Autodesk Inventor part; units mm, degrees
ref_plane "作業平面1" through (28.1996, -140.8267, 0) normal (-1, 0, 0) x (0, 0, 1)
ref_plane "作業平面2" through (-116.8004, -45.8267, 0) normal (0, 1, 0) x (1, 0, 0)
ref_plane "YZ Plane" through (0, 0, 0) normal (1, 0, 0) x (0, 1, 0)
sketch "スケッチ1" plane through (0, 0, 0) normal (0, 0, 1) x (1, 0, 0)
  line L0 (-116.8004, 49.1733) -> (173.1996, 49.1733)
  line L1 (173.1996, 49.1733) -> (173.1996, -140.8267)
  line L2 (173.1996, -140.8267) -> (-116.8004, -140.8267)
  line L3 (-116.8004, -140.8267) -> (-116.8004, 49.1733)
  point P0 (0, 0)
  dimension "d0" = 290
  dimension "d1" = 190
extrude "押し出し1" add sketch "スケッチ1" along normal blind 15
sketch "スケッチ2" plane through (0, 0, 15) normal (0, 0, 1) x (1, 0, 0)
  line L0 (-111.8004, 42.1733) -> (163.1996, 42.1733)
  line L1 (163.1996, 42.1733) -> (163.1996, -133.8267)
  line L2 (163.1996, -133.8267) -> (-111.8004, -133.8267)
  line L3 (-111.8004, -133.8267) -> (-111.8004, 42.1733)
  line L4 (-111.8004, 27.1733) -> (-99.8004, 27.1733)
  line L5 (-99.8004, 27.1733) -> (-99.8004, 42.1733)
  line L6 (-116.8004, 49.1733) -> (-116.8004, -140.8267)
  line L7 (-116.8004, -140.8267) -> (173.1996, -140.8267)
  line L8 (173.1996, 49.1733) -> (-116.8004, 49.1733)
  line L9 (28.1996, -45.8267) -> (-116.8004, -45.8267)
  line L10 (28.1996, -45.8267) -> (28.1996, 49.1733)
  line L11 (168.1996, 27.1733) -> (158.1996, 27.1733)
  line L12 (158.1996, 27.1733) -> (158.1996, 42.1733)
  line L13 (-111.8004, -118.8267) -> (-99.8004, -118.8267)
  line L14 (-99.8004, -118.8267) -> (-99.8004, -133.8267)
  line L15 (158.1996, -118.8267) -> (158.1996, -133.8267)
  line L16 (168.1996, -118.8267) -> (158.1996, -118.8267)
  line L17 (-99.8004, 27.1733) -> (-99.8004, -118.8267)
  line L18 (158.1996, 27.1733) -> (151.1996, 27.1733)
  line L19 (151.1996, 27.1733) -> (151.1996, 42.1733)
  line L20 (158.1996, -118.8267) -> (151.1996, -118.8267)
  line L21 (151.1996, -118.8267) -> (151.1996, -133.8267)
  point P0 (0, 0)
  point P1 (163.1996, -118.8267)
  point P2 (163.1996, 27.1733)
  point P3 (158.1996, 42.1733)
  point P4 (-111.8004, -118.8267)
  point P5 (158.1996, -133.8267)
  dimension "d4" = 15
  dimension "d5" = 275
  dimension "d6" = 5
  dimension "d7" = 7
  dimension "d8" = 7
  dimension "d9" = 12
  dimension "d15" = 7
ref_plane "作業平面1" through (28.1996, -140.8267, 0) normal (-1, 0, 0) x (0, 0, 1)
ref_plane "作業平面2" through (-116.8004, -45.8267, 0) normal (0, 1, 0) x (1, 0, 0)
extrude "押し出し2" cut sketch "スケッチ2" against normal blind 8 contours L0 L10 L9 L17 L5 | L0 L19 L18 L11 L1 L16 L20 L21 L2 L14 L17 L9 L10 | L21 L20 L15 L2
sketch "スケッチ3" plane through (-116.8004, -140.8267, 0) normal (0, -1, 0) x (1, 0, 0)
  line L0 (275, 15) -> (275, 7)
  line L1 (275, 7) -> (17, 7)
  line L2 (275, 7) -> (270, 7)
  line L3 (270, 7) -> (270, 15)
  line L4 (0, 15) -> (290, 15)
  line L5 (270, 7) -> (270, 0)
  line L6 (290, 0) -> (0, 0)
  line L7 (275, 15) -> (275, 7)
  line L8 (275, 0) -> (275, 7)
  point P0 (116.8004, 0)
  dimension "d12" = 5
extrude "押し出し3" cut sketch "スケッチ3" against normal blind 7
sketch "スケッチ4" plane through (0, 0, 15) normal (0, 0, 1) x (1, 0, 0)
  circle A0 centre (-106.8004, 39.1733) radius 2.25
  circle A1 centre (163.1996, 39.1733) radius 2.25
  circle A2 centre (163.1996, -130.8267) radius 2.25
  line L0 (153.1996, -133.8267) -> (-99.8004, -133.8267)
  line L1 (-99.8004, -133.8267) -> (-99.8004, 42.1733)
  line L2 (-99.8004, 42.1733) -> (151.1996, 42.1733)
  line L3 (151.1996, 42.1733) -> (151.1996, 27.1733)
  line L4 (151.1996, 27.1733) -> (163.1996, 27.1733)
  line L5 (163.1996, 27.1733) -> (163.1996, -118.8267)
  line L6 (163.1996, -118.8267) -> (158.1996, -118.8267)
  line L7 (158.1996, -118.8267) -> (158.1996, -140.8267)
  line L8 (-116.8004, -140.8267) -> (153.1996, -140.8267)
  line L9 (173.1996, -140.8267) -> (173.1996, 49.1733)
  line L10 (173.1996, 49.1733) -> (-116.8004, 49.1733)
  line L11 (-116.8004, 49.1733) -> (-116.8004, -140.8267)
  line L12 (158.1996, -140.8267) -> (173.1996, -140.8267)
  circle A3 centre (-106.8004, -130.8267) radius 2.25
  line L13 (153.1996, -140.8267) -> (153.1996, -133.8267)
  point P0 (0, 0)
hole "穴1" at (-106.8004, 39.1733, 15) at (-106.8004, -130.8267, 15) at (163.1996, -130.8267, 15) at (163.1996, 39.1733, 15) direction (0, 0, -1) diameter 4.2 depth 4
fillet "フィレット2" radius 7 3 edges at (-99.8004, 42.1733, 11) (-99.8004, -133.8267, 11) (151.1996, 42.1733, 11)
fillet "フィレット3" radius 5 4 edges at (151.1996, 27.1733, 11) (163.1996, 27.1733, 11) (158.1996, -118.8267, 11) (163.1996, -118.8267, 11)
sketch "スケッチ5" plane through (0, 0, 0) normal (0, 0, -1) x (-1, 0, 0)
  line L0 (-143.1996, 41.1733) -> (92.8004, 41.1733)
  line L1 (92.8004, -133.8267) -> (-143.1996, -133.8267)
  line L2 (99.8004, 34.1733) -> (99.8004, -126.8267)
  line L3 (-163.1996, 22.1733) -> (-163.1996, -113.8267)
  line L4 (-173.1996, -140.8267) -> (-173.1996, 49.1733)
  line L5 (-28.1996, 87.1733) -> (-28.1996, -178.8267)
  line L6 (-231.1996, -45.8267) -> (174.8004, -45.8267)
  line L7 (-173.1996, 49.1733) -> (116.8004, 49.1733)
  point P0 (0, 0)
  point P1 (-98.1996, 41.6733)
  point P2 (41.8004, 41.6733)
  point P3 (-98.1996, -133.3267)
  point P4 (41.8004, -133.3267)
  point P5 (-165.6996, -30.8267)
  point P6 (-165.6996, -60.8267)
  point P7 (109.3004, -30.8267)
  point P8 (109.3004, -60.8267)
  point P9 (-68.1996, 41.6733)
  point P10 (11.8004, 41.6733)
  point P11 (-68.1996, -133.3267)
  point P12 (11.8004, -133.3267)
  dimension "d26" = 75
  dimension "d27" = 7.5
  dimension "d28" = 15
  dimension "d29" = 7.5
  dimension "d30" = 30
  dimension "d31" = 7.5
hole "穴2" at (98.1996, 41.6733, 0) at (-41.8004, 41.6733, 0) at (98.1996, -133.3267, 0) at (-41.8004, -133.3267, 0) at (165.6996, -30.8267, 0) at (165.6996, -60.8267, 0) at (-109.3004, -30.8267, 0) at (-109.3004, -60.8267, 0) at (68.1996, 41.6733, 0) at (-11.8004, 41.6733, 0) at (68.1996, -133.3267, 0) at (-11.8004, -133.3267, 0) direction (0, 0, 1) diameter 4.2 depth 4
properties part number "iPadHolder"
For this review, take the finished solid that the model builds, in its own axes (mm). A direction names the side the tool comes from. Give positions to 0.01 mm unless a question says otherwise; leave off trailing zeros. Write each loop counter-clockwise with the first axis right and the second up, starting at its lowest first coordinate (ties: lowest second). Pieces come first, ordered by that corner, then holes. Notation, with made-up numbers: M 86.25,-5 L 123.25,-5 A16 cw 123.25,7 Z; hole C -13,33 d5. An arc over 180 degrees is marked long. Answer as a JSON object with one key per item and string values. Group by question number.
Item 1: Draft analysis for pull direction X (two halves, no side actions). For faces 1 (the flat face through (-116.8, -47, 7)), 2 (the flat face through (26, -44, 0)), 3 (the flat face through (153.2, -137, 7)), state which applies: +X half, -X half, draft (parallel to the pull), parting line (faces both ways), or undercut.
Item 2: Tool access review of faces 4 (the flat face through (32, -133.827, 11)), 5 (the flat face through (158.2, -134, 9)), 6 (the flat face through (6, 46, 15)): name each direction out of +Z, -Z, +X, -X, +Y, -Y from which nothing blocks a thin tool from reaching the whole face with its end or side.
Item 3: For probe 1 along Y at (x, z) = (-42, 13); probe 2 along X at (y, z) = (6, 9.25); probe 3 along Y at (x, z) = (66.5, 3.25), list the stretches that pass through material, from the lowest coordinate up. Write a range as [from, to].
Item 4: Consider section A-A on x = 15. Write out the cut boundary in (y, z), plus the area to 3 significant figures.
Item 5: For pin 1 Ø4 at (x, y) = (65, -6) entering from -Z; pin 2 Ø3.5 at (x, y) = (98.2, -133.33) entering from -Z; pin 3 Ø8 at (x, y) = (-73.5, -85.5) entering from +Z; pin 4 Ø2 at (x, y) = (-107, 39.5) entering from +Z, all flat-tipped, find the tip position at first contact; note any pin that passes through.
Item 6: Consider section B-B on y = -21.5. Write out the cut boundary in (x, z), plus the area to 3 significant figures.
Check result:
{
 "1": {"face 1": "-X half", "face 2": "draft", "face 3": "undercut"},
 "2": {"face 4": "+Z", "face 5": "+Z, -Y", "face 6": "+Z, +X, -X, +Y, -Y"},
 "3": {"probe 1": "y = [-140.83, -133.83], [42.17, 49.17]", "probe 2": "x = [-116.8, -99.8], [163.2, 173.2]", "probe 3": "y = [-140.83, -134.56], [-132.09, 40.44], [42.91, 49.17]"},
 "4": {"outline": "M -140.83,0 L 49.17,0 L 49.17,15 L 42.17,15 L 42.17,7 L -133.83,7 L -133.83,15 L -140.83,15 Z", "area": "1,440 mm^2"},
 "5": {"pin 1": "stops at z = 0", "pin 2": "stops at z = 4", "pin 3": "stops at z = 7", "pin 4": "stops at z = 11"},
 "6": {"outline": "M -116.8,0 L 173.2,0 L 173.2,15 L 163.2,15 L 163.2,7 L -99.8,7 L -99.8,15 L -116.8,15 Z", "area": "2,250 mm^2"}
}
